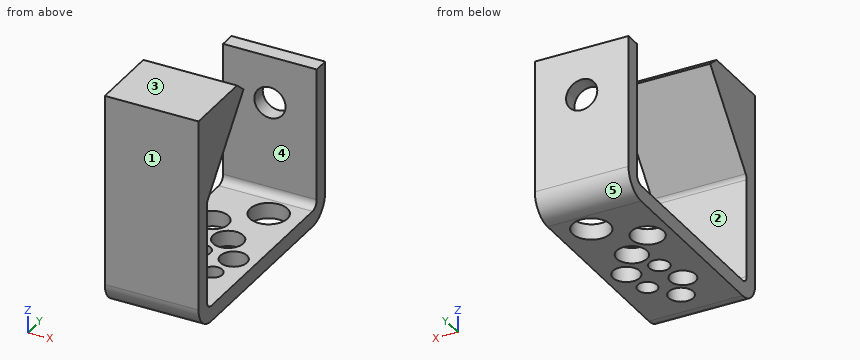
from build123d import *

# Parameters (mm, degrees)
BASE_EXTRUDE_THIN_DEPTH = 19.05
CUT_EXTRUDE1_REACH      = 97.25
SKETCH2_R               = 6.35
BOSS_EXTRUDE1_START     = -19.05
BOSS_EXTRUDE1_DEPTH     = 38.1
CUT_EXTRUDE2_REACH      = 89.648
SKETCH4_R               = 7.602418737
SKETCH4_R_2             = 6.149803706
SKETCH4_R_3             = 6.52839763
SKETCH4_R_4             = 4.086633044
SKETCH4_R_5             = 3.965992325
SKETCH4_R_6             = 5.18600248
SKETCH4_R_7             = 4.976076495
SKETCH4_R_8             = 5.4229927


with BuildPart() as part:
    # Sketch1 → Base-Extrude-Thin (new body, symmetric)
    with BuildSketch(Plane(origin=(0, 0, 0), x_dir=(0, 0, -1), z_dir=(1, 0, 0))):
        with BuildLine():
            Line((-77.216478592, 27.494340102), (-45.335245167, 0.742808893))
            ThreePointArc((-45.335245167, 0.742808893), (-44.380308461, 0.191475929), (-43.294394506, 0))
            Line((-43.294394506, 0), (-3.175, 0))
            ThreePointArc((-3.175, 0), (-0.92993597, 0.92993597), (0, 3.175))
            Line((0, 3.175), (0, 79.375))
            ThreePointArc((0, 79.375), (-0.92993597, 81.62006403), (-3.175, 82.55))
            Line((-3.175, 82.55), (-57.15, 82.55))
            Line((-57.15, 82.55), (-57.15, 88.9))
            Line((-57.15, 88.9), (-3.175, 88.9))
            ThreePointArc((-3.175, 88.9), (3.560192091, 86.110192091), (6.35, 79.375))
            Line((6.35, 79.375), (6.35, 3.175))
            ThreePointArc((6.35, 3.175), (3.560192091, -3.560192091), (-3.175, -6.35))
            Line((-3.175, -6.35), (-43.294394506, -6.35))
            ThreePointArc((-43.294394506, -6.35), (-46.552136371, -5.775572213), (-49.416946488, -4.121573321))
            Line((-49.416946488, -4.121573321), (-81.298179914, 22.629957888))
            Line((-81.298179914, 22.629957888), (-77.216478592, 27.494340102))
        make_face()
    extrude(amount=BASE_EXTRUDE_THIN_DEPTH, both=True)

    # Sketch2 → Cut-Extrude1 (cut, up to next)
    with BuildSketch(Plane(origin=(0, 88.9, 0), x_dir=(-1, 0, 0), z_dir=(0, 1, 0)), mode=Mode.PRIVATE) as cut_extrude1_sk1:
        with Locations((0, 38.1)):
            Circle(SKETCH2_R)
    cut_extrude1_tool1 = extrude(cut_extrude1_sk1.sketch, amount=-CUT_EXTRUDE1_REACH, mode=Mode.PRIVATE) & part.part
    add(cut_extrude1_tool1.solids().sort_by_distance((0, 88.9, 38.1))[0], mode=Mode.SUBTRACT)

    # Sketch3 → Boss-Extrude1 (add)
    with BuildSketch(Plane(origin=(0, 0, 0), x_dir=(0, 0, -1), z_dir=(1, 0, 0)).offset(BOSS_EXTRUDE1_START)):
        with BuildLine():
            Line((-49.416946488, -4.121573321), (-81.298179914, 22.629957888))
            Line((-81.298179914, 22.629957888), (-81.298179914, -6.35))
            Line((-81.298179914, -6.35), (-43.294394506, -6.35))
            ThreePointArc((-43.294394506, -6.35), (-46.552136371, -5.775572213), (-49.416946488, -4.121573321))
        make_face()
    extrude(amount=BOSS_EXTRUDE1_DEPTH)

    # Sketch4 → Cut-Extrude2 (cut, up to next)
    with BuildSketch(Plane(origin=(0, 0, -6.35), x_dir=(-1, 0, 0), z_dir=(0, 0, -1)), mode=Mode.PRIVATE) as cut_extrude2_sk1:
        with Locations((-6.048622008, 70.468859283)):
            Circle(SKETCH4_R)
    cut_extrude2_tool1 = extrude(cut_extrude2_sk1.sketch, amount=-CUT_EXTRUDE2_REACH, mode=Mode.PRIVATE) & part.part
    add(cut_extrude2_tool1.solids().sort_by_distance((6.048622, 70.468859, -6.35))[0], mode=Mode.SUBTRACT)
    # Sketch4 → Cut-Extrude2 (cut, up to next)
    with BuildSketch(Plane(origin=(0, 0, -6.35), x_dir=(-1, 0, 0), z_dir=(0, 0, -1)), mode=Mode.PRIVATE) as cut_extrude2_sk2:
        with Locations((-1.975060247, 47.508783906)):
            Circle(SKETCH4_R_2)
    cut_extrude2_tool2 = extrude(cut_extrude2_sk2.sketch, amount=-CUT_EXTRUDE2_REACH, mode=Mode.PRIVATE) & part.part
    add(cut_extrude2_tool2.solids().sort_by_distance((1.97506, 47.508784, -6.35))[0], mode=Mode.SUBTRACT)
    # Sketch4 → Cut-Extrude2 (cut, up to next)
    with BuildSketch(Plane(origin=(0, 0, -6.35), x_dir=(-1, 0, 0), z_dir=(0, 0, -1)), mode=Mode.PRIVATE) as cut_extrude2_sk3:
        with Locations((9.504977441, 56.890320082)):
            Circle(SKETCH4_R_3)
    cut_extrude2_tool3 = extrude(cut_extrude2_sk3.sketch, amount=-CUT_EXTRUDE2_REACH, mode=Mode.PRIVATE) & part.part
    add(cut_extrude2_tool3.solids().sort_by_distance((-9.504977, 56.89032, -6.35))[0], mode=Mode.SUBTRACT)
    # Sketch4 → Cut-Extrude2 (cut, up to next)
    with BuildSketch(Plane(origin=(0, 0, -6.35), x_dir=(-1, 0, 0), z_dir=(0, 0, -1)), mode=Mode.PRIVATE) as cut_extrude2_sk4:
        with Locations((3.086031637, 36.152187483)):
            Circle(SKETCH4_R_4)
    cut_extrude2_tool4 = extrude(cut_extrude2_sk4.sketch, amount=-CUT_EXTRUDE2_REACH, mode=Mode.PRIVATE) & part.part
    add(cut_extrude2_tool4.solids().sort_by_distance((-3.086032, 36.152187, -6.35))[0], mode=Mode.SUBTRACT)
    # Sketch4 → Cut-Extrude2 (cut, up to next)
    with BuildSketch(Plane(origin=(0, 0, -6.35), x_dir=(-1, 0, 0), z_dir=(0, 0, -1)), mode=Mode.PRIVATE) as cut_extrude2_sk5:
        with Locations((-8.124863953, 24.425267264)):
            Circle(SKETCH4_R_5)
    cut_extrude2_tool5 = extrude(cut_extrude2_sk5.sketch, amount=-CUT_EXTRUDE2_REACH, mode=Mode.PRIVATE) & part.part
    add(cut_extrude2_tool5.solids().sort_by_distance((8.124864, 24.425267, -6.35))[0], mode=Mode.SUBTRACT)
    # Sketch4 → Cut-Extrude2 (cut, up to next)
    with BuildSketch(Plane(origin=(0, 0, -6.35), x_dir=(-1, 0, 0), z_dir=(0, 0, -1)), mode=Mode.PRIVATE) as cut_extrude2_sk6:
        with Locations((6.295504539, 24.425267264)):
            Circle(SKETCH4_R_6)
    cut_extrude2_tool6 = extrude(cut_extrude2_sk6.sketch, amount=-CUT_EXTRUDE2_REACH, mode=Mode.PRIVATE) & part.part
    add(cut_extrude2_tool6.solids().sort_by_distance((-6.295505, 24.425267, -6.35))[0], mode=Mode.SUBTRACT)
    # Sketch4 → Cut-Extrude2 (cut, up to next)
    with BuildSketch(Plane(origin=(0, 0, -6.35), x_dir=(-1, 0, 0), z_dir=(0, 0, -1)), mode=Mode.PRIVATE) as cut_extrude2_sk7:
        with Locations((0, 14.17964223)):
            Circle(SKETCH4_R_7)
    cut_extrude2_tool7 = extrude(cut_extrude2_sk7.sketch, amount=-CUT_EXTRUDE2_REACH, mode=Mode.PRIVATE) & part.part
    add(cut_extrude2_tool7.solids().sort_by_distance((0, 14.179642, -6.35))[0], mode=Mode.SUBTRACT)
    # Sketch4 → Cut-Extrude2 (cut, up to next)
    with BuildSketch(Plane(origin=(0, 0, -6.35), x_dir=(-1, 0, 0), z_dir=(0, 0, -1)), mode=Mode.PRIVATE) as cut_extrude2_sk8:
        with Locations((-10.369066299, 36.152187483)):
            Circle(SKETCH4_R_8)
    cut_extrude2_tool8 = extrude(cut_extrude2_sk8.sketch, amount=-CUT_EXTRUDE2_REACH, mode=Mode.PRIVATE) & part.part
    add(cut_extrude2_tool8.solids().sort_by_distance((10.369066, 36.152187, -6.35))[0], mode=Mode.SUBTRACT)


solid = part.part
The listing builds one solid part. Answer for the finished solid, in the listing's coordinates (mm). Face numbers are marked on the shaded views. A direction names the side the tool comes from. Round coordinates to 2 decimals unless told otherwise and drop trailing zeros. Order: outer loops, then holes, each group sorted by start corner. A loop starts at its lowest first (then second) coordinate and runs counter-clockwise, first axis right, second up. Notation, with made-up numbers: (51.25, 33) -> (94.25, 33) arc R24 ccw to (94.25, 58) -> close; hole circle Ø8 at (68.5, 56). An arc over 180 degrees is marked (long way). Put each result on its own line as item: value.
Q1. Section D-D, the plane y = 12 is taken. Write down the section's boundary in (x, z).
Results list:
outline: (-19.05, -6.35) -> (-4.47, -6.35) -> (-4.47, 0) -> (-19.05, 0) -> close; (-19.05, 58.75) -> (19.05, 58.75) -> (19.05, 81.3) -> (-19.05, 81.3) -> close; (4.47, -6.35) -> (19.05, -6.35) -> (19.05, 0) -> (4.47, 0) -> close
Q2. Determine the mould class of the marked faces 3, 4 and 5 for opening direction Y: pulls with the +Y half, pulls with the -Y half, needs draft (parallel to the pull), parting line crosses it, or undercut.
Results list:
face 3: needs draft
face 4: undercut
face 5: pulls with the +Y half
Q3. Section A-A, the plane z = 38.1 is taken. Write down the section's boundary in (x, y), and give its area (3 significant figures).
Results list:
outline: (-19.05, -6.35) -> (19.05, -6.35) -> (19.05, 0) -> (-19.05, 0) -> close; (-19.05, 82.55) -> (-6.35, 82.55) -> (-6.35, 88.9) -> (-19.05, 88.9) -> close; (6.35, 82.55) -> (19.05, 82.55) -> (19.05, 88.9) -> (6.35, 88.9) -> close
area: 403 mm^2
Q4. Which of the six approach directions +Z, -Z, +X, -X, +Y, -Y give full straight-line access (tool end or side, diameter ignored) to the marked faces 1 and 2?
Results list:
face 1: +Z, -Z, +X, -X, -Y
face 2: +X, -X
Q5. Each of these flat-tipped pins is pushed along its axis until it touches: P1, Ø9.5, axis at x = -6.3, y = 24.43, coming from the +Z side; P2, Ø1, axis at x = 4.5, y = 39.5, coming from the +Z side; P3, Ø10, axis at x = 0, z = 38.1, coming from the +Y side; P4, Ø5, axis at x = 8, y = 86.5, coming from the +Z side. Where does it stop, or does it pass through?
Results list:
P1: z = 81.3
P2: z = 0
P3: y = 0
P4: z = 57.15
Q6. Section C-C, the plane z = 4.5 is taken. Write down the section's boundary in (x, y).
Results list:
outline: (-19.05, -6.35) -> (19.05, -6.35) -> (19.05, 0) -> (-19.05, 0) -> close; (-19.05, 82.55) -> (19.05, 82.55) -> (19.05, 88.9) -> (-19.05, 88.9) -> close
Q7. Consider line 1 along Y through (x, z) = (-2.5, 22); line 2 along Y through (x, z) = (0, -2.75); line 3 along Y through (x, z) = (0, -2). Determine where each line is inside the solid, lowest interval first.
Results list:
line 1: -6.35 to 0, 82.55 to 88.9
line 2: -4.28 to 9.2, 19.16 to 33.47, 38.83 to 41.68, 53.33 to 65.86, 75.07 to 86.83
line 3: -4.82 to 9.2, 19.16 to 33.47, 38.83 to 41.68, 53.33 to 65.86, 75.07 to 87.37
Q8. Section B-B, the plane y = 58.5 is taken. Write down the section's boundary in (x, z).
Results list:
outline: (-19.05, -6.35) -> (-15.83, -6.35) -> (-15.83, 0) -> (-19.05, 0) -> close; (-3.18, -6.35) -> (19.05, -6.35) -> (19.05, 0) -> (-3.18, 0) -> close
